CAD build for the part. Positions are in the model's coordinates, mm. A direction names the side the tool comes from. Coordinates: 2 decimals unless noted, no trailing zeros. Loops run counter-clockwise (first coordinate to the right, second up) from the corner with the lowest first, then second, coordinate; pieces in that order, holes last. Notation, with made-up numbers: (57, 6.5) -> (81, 6.5) arc R33 cw to (81, 34.5) -> close; hole circle Ø2 at (55.5, 35). An arc over 180 degrees is marked (long way). Write item = value, one per line. Start each with the question number.
(1) Band-saw the part on D-D (x = -3.75). Count the separate pieces of the cut face and the enclosed holes in it, and give its area (3 significant figures).
(2) Tool access for faces 3 (the face through (-3, -3.33, -1)), 4 (the face through (-3, 3, -8.575)), 5 (the face through (-3, 12, -19.137)): list every direction of +Z, -Z, +X, -X, +Y, -Y with a clear straight run to the whole face (end or side of a thin tool).
(3) Band-saw the part on B-B (y = 25.15). Write the cut outline in (x, z) (3 decimals), and give its area (3 significant figures).
(4) Band-saw the part on C-C (x = -7.62). Write the cut outline in (y, z) (3 decimals), and give its area (4 significant figures).
(5) Band-saw the part on A-A (z = -27.23). Write the cut outline in (x, y) (3 decimals), and give its area (3 significant figures).
(6) Pull direction Z, two halves, no side cores. Call faces 1 (the face through (-3, 9, -4.75)), 2 (the face through (-1.73, 25, -8)): +Z half, -Z half, draft (parallel to the pull), parting line (faces both ways), or undercut.
(7) Flat gauge pins, fed straight in: P1, Ø1, axis at x = -1.5, y = 3, coming from the -Z side; P2, Ø1.5, axis at x = -2.5, z = -24, coming from the +Y side; P3, Ø1.3, axis at x = -1.5, z = -9.5, coming from the -Y side. Where does each tip first touch, or does it go through?
(8) Drill centre lines: line 1 (Y direction, x = -2.25, z = -3) (3 decimals); line 2 (Z direction, x = -7.62, y = 0.75) (3 decimals); line 3 (Y direction, x = -4.5, z = -22). Where is each one in solid material? Low to high. Write a range as from..to.
```python
from build123d import *

# Parameters (mm, degrees)
BOSS_EXTRUDE1_DEPTH = 5.18
CUT_EXTRUDE4_REACH  = 42.076
SKETCH2_W           = 3.45
SKETCH2_H           = 5.15
CUT_EXTRUDE3_REACH  = 43.319
SKETCH7_R           = 1.575
SKETCH3_W           = 10.5
SKETCH3_H           = 30
SKETCH3_R           = 1.575
BOSS_EXTRUDE2_DEPTH = 1.5


with BuildPart() as part:
    # Sketch1 → Boss-Extrude1 (new body)
    with BuildSketch(Plane(origin=(0, 0, 0), x_dir=(0, 0, -1), z_dir=(1, 0, 0))):
        Polygon((2, 29.025), (2, 21.375), (13.75, 21.375), (13.75, 20.033333333), (11.75, 20.033333333), (11.75, 20.208333333), (5.25, 20.208333333), (5.25, 20.033333333), (3.25, 20.033333333), (3.25, 20.208333333), (2, 20.208333333), (2, 15.958333333), (3.25, 15.958333333), (3.25, 16.133333333), (5.25, 16.133333333), (5.25, 15.958333333), (11.75, 15.958333333), (11.75, 16.133333333), (13.75, 16.133333333), (13.75, 15.738333333), (2, 15.738333333), (2, 14.488333333), (2.175, 14.488333333), (2.175, 12.488333333), (2, 12.488333333), (2, 4.5), (2.175, 4.5), (2.175, 2.5), (0, 2.5), (-1.5, 1), (-1.5, -4.83), (2.5, -4.83), (2.5, -3.33), (0, -3.33), (0, 0), (26.303333333, 0), (24.553333333, 12.1875), (20.886666667, 12.1875), (20.886666667, 10.9375), (21.061666667, 10.9375), (21.061666667, 8.9375), (20.886666667, 8.9375), (20.886666667, 6.25), (21.061666667, 6.25), (21.061666667, 4.25), (18.961666667, 4.25), (18.961666667, 6.25), (19.136666667, 6.25), (19.136666667, 18.125), (18.961666667, 18.125), (18.961666667, 20.125), (19.136666667, 20.125), (19.136666667, 21.375), (16.72, 21.375), (16.72, 31.441666667), (13.75, 31.441666667), (13.75, 31.116666667), (11.75, 31.116666667), (11.75, 31.441666667), (7.75, 31.441666667), (7.75, 31.116666667), (5.75, 31.116666667), (5.75, 31.441666667), (4.5, 31.441666667), (4.5, 29.025), align=None)
        Polygon((5.75, 29.025), (15, 29.025), (15, 18.958333333), (13.75, 18.958333333), (13.75, 19.133333333), (11.75, 19.133333333), (11.75, 18.958333333), (5.25, 18.958333333), (5.25, 19.133333333), (3.25, 19.133333333), (3.25, 17.033333333), (5.25, 17.033333333), (5.25, 17.208333333), (11.75, 17.208333333), (11.75, 17.033333333), (13.75, 17.033333333), (13.75, 17.208333333), (15, 17.208333333), (15, 15.738333333), (15.22, 15.738333333), (15.22, 30.191666667), (13.75, 30.191666667), (13.75, 30.366666667), (11.75, 30.366666667), (11.75, 30.191666667), (7.75, 30.191666667), (7.75, 30.366666667), (5.75, 30.366666667), align=None, mode=Mode.SUBTRACT)
        Polygon((18.061666667, 4.25), (17.886666667, 4.25), (17.886666667, 3), (22.136666667, 3), (22.136666667, 4.25), (21.961666667, 4.25), (21.961666667, 6.25), (22.136666667, 6.25), (22.136666667, 8.9375), (21.961666667, 8.9375), (21.961666667, 10.9375), (23.303333333, 10.9375), (23.303333333, 2.5), (8.575, 2.5), (8.575, 4.5), (8.75, 4.5), (8.75, 12.488333333), (8.575, 12.488333333), (8.575, 14.488333333), (10.25, 14.488333333), (10.25, 3), (16.72, 3), (16.72, 20.125), (18.061666667, 20.125), (18.061666667, 18.125), (17.886666667, 18.125), (17.886666667, 6.25), (18.061666667, 6.25), align=None, mode=Mode.SUBTRACT)
        Polygon((3.075, 2.5), (3.075, 4.5), (3.25, 4.5), (3.25, 12.488333333), (3.075, 12.488333333), (3.075, 14.488333333), (4.925, 14.488333333), (4.925, 12.488333333), (4.75, 12.488333333), (4.75, 4.5), (4.925, 4.5), (4.925, 2.5), align=None, mode=Mode.SUBTRACT)
        Polygon((5.825, 2.5), (5.825, 4.5), (6, 4.5), (6, 12.488333333), (5.825, 12.488333333), (5.825, 14.488333333), (7.675, 14.488333333), (7.675, 12.488333333), (7.5, 12.488333333), (7.5, 4.5), (7.675, 4.5), (7.675, 2.5), align=None, mode=Mode.SUBTRACT)
    extrude(amount=BOSS_EXTRUDE1_DEPTH)

    # Sketch2 → Cut-Extrude4 (cut, up to next)
    with BuildSketch(Plane.XY.offset(-2), mode=Mode.PRIVATE) as cut_extrude4_sk1:
        with Locations((3.455, 25.2)):
            Rectangle(SKETCH2_W, SKETCH2_H)
    cut_extrude4_tool1 = extrude(cut_extrude4_sk1.sketch, amount=-CUT_EXTRUDE4_REACH, mode=Mode.PRIVATE) & part.part
    add(cut_extrude4_tool1.solids().sort_by_distance((3.455, 25.2, -2))[0], mode=Mode.SUBTRACT)

    # Sketch7 → Cut-Extrude3 (cut, up to next)
    with BuildSketch(Plane.ZY, mode=Mode.PRIVATE) as cut_extrude3_sk1:
        with Locations((-5.25, 25.15)):
            Circle(SKETCH7_R)
    cut_extrude3_tool1 = extrude(cut_extrude3_sk1.sketch, amount=-CUT_EXTRUDE3_REACH, mode=Mode.PRIVATE) & part.part
    # Sketch7 → Cut-Extrude3 (cut, up to next)
    with BuildSketch(Plane.ZY, mode=Mode.PRIVATE) as cut_extrude3_sk2:
        with Locations((-11.75, 25.15)):
            Circle(SKETCH7_R)
    cut_extrude3_tool2 = extrude(cut_extrude3_sk2.sketch, amount=-CUT_EXTRUDE3_REACH, mode=Mode.PRIVATE) & part.part
    add(cut_extrude3_tool1.solids().sort_by_distance((0, 25.15, -5.25))[0], mode=Mode.SUBTRACT)
    add(cut_extrude3_tool2.solids().sort_by_distance((0, 25.15, -11.75))[0], mode=Mode.SUBTRACT)

    # Sketch3 → Boss-Extrude2 (add)
    with BuildSketch(Plane.XZ):
        with Locations((5.25, -15)):
            Rectangle(SKETCH3_W, SKETCH3_H)
        with Locations(Location((7.62, -15.23, 0), (0, 0, 270))):
            Circle(SKETCH3_R, mode=Mode.SUBTRACT)
        with Locations(Location((7.62, -27.23, 0), (0, 0, 270))):
            Circle(SKETCH3_R, mode=Mode.SUBTRACT)
    extrude(amount=-BOSS_EXTRUDE2_DEPTH)


with BuildPart() as body_2:
    # Mirror1: mirrored copy
    add(part.part.mirror(Plane.ZY))


solid = body_2.part
```
Findings below:
q1.separate_pieces = 1
q1.enclosed_holes = 3
q1.area = 376 mm²
q2.face_3 = -Z, +X, -X
q2.face_4 = +X, -X
q2.face_5 = +X, -X, +Y
q3.outline = (-5.18, -16.72) -> (0, -16.72) -> (0, -15.22) -> (-5.18, -15.22) -> close; (-1.73, -15) -> (0, -15) -> (0, -13.325) -> (-1.73, -13.325) -> close; (-1.73, -10.175) -> (0, -10.175) -> (0, -6.825) -> (-1.73, -6.825) -> close; (-1.73, -3.675) -> (0, -3.675) -> (0, -2) -> (-1.73, -2) -> close
q3.area = 19.4 mm²
q4.outline = (0, -30) -> (1.5, -30) -> (1.5, -28.805) -> (0, -28.805) -> close; (0, -25.655) -> (1.5, -25.655) -> (1.5, -16.805) -> (0, -16.805) -> close; (0, -13.655) -> (1.5, -13.655) -> (1.5, 0) -> (0, 0) -> close
q4.area = 35.55 mm²
q5.outline = (-10.5, 0) -> (-9.195, 0) -> (-9.195, 1.5) -> (-10.5, 1.5) -> close; (-6.045, 0) -> (0, 0) -> (0, 1.5) -> (-6.045, 1.5) -> close
q5.area = 11.0 mm²
q6.face_1 = undercut
q6.face_2 = draft
q7.P1 = -25.94
q7.P2 = 12.19
q7.P3 = 0
q8.line_1 = 0..15.738, 15.958..20.208, 21.375..22.625, 27.775..29.025
q8.line_2 = -30..-28.805, -25.655..-16.805, -13.655..0
q8.line_3 = 0..2.5, 3..4.25, 6.25..8.94, 10.94..12.19
